from build123d import *

# Parameters (mm, degrees)
SKETCH1_R           = 2
BOSS_EXTRUDE1_DEPTH = 2


with BuildPart() as part:
    # Sketch1 → Boss-Extrude1 (new body)
    with BuildSketch(Plane.XY):
        with BuildLine():
            Line((43.801010204, 68), (43.801010204, 71.053350769))
            ThreePointArc((43.801010204, 71.053350769), (45.533161176, 74.837681982), (49.529475295, 76))
            ThreePointArc((49.529475295, 76), (115.157062367, 0), (49.529475295, -76))
            ThreePointArc((49.529475295, -76), (45.533161176, -74.837681982), (43.801010204, -71.053350769))
            Line((43.801010204, -71.053350769), (43.801010204, -68))
            ThreePointArc((43.801010204, -68), (40.286291578, -59.514718626), (31.801010204, -56))
            Line((31.801010204, -56), (-106.198989796, -56))
            ThreePointArc((-106.198989796, -56), (-126.131547425, 0), (-106.198989796, 56))
            Line((-106.198989796, 56), (31.801010204, 56))
            ThreePointArc((31.801010204, 56), (40.286291578, 59.514718626), (43.801010204, 68))
        make_face()
        with Locations((67, 44)):
            Circle(SKETCH1_R, mode=Mode.SUBTRACT)
        with Locations((67, -44)):
            Circle(SKETCH1_R, mode=Mode.SUBTRACT)
        with Locations((-67, 44)):
            Circle(SKETCH1_R, mode=Mode.SUBTRACT)
        with Locations((-67, -44)):
            Circle(SKETCH1_R, mode=Mode.SUBTRACT)
    extrude(amount=BOSS_EXTRUDE1_DEPTH)


solid = part.part
Build history of the part. All positions in model axes, mm. Coordinates: 2 decimals unless noted, no trailing zeros. Order: outer loops, then holes, each group sorted by start corner. A loop starts at its lowest first (then second) coordinate and runs counter-clockwise, first axis right, second up. Notation, with made-up numbers: (75.5, 64) - (83.5, 64) arc R9 cw to (83.5, 78) - close; hole circle Ø10 at (12.25, -32). An arc over 180 degrees is marked (long way). Write each question's results on one line, items separated by ' | '. Start each with the question number.
Item 1: Band-saw the part on A-A on z = 1.7. Write the cut outline in (x, y).
Item 2: Band-saw the part on C-C on y = 26. Write the cut outline in (x, z).
Item 3: Flat gauge pins, fed straight in: pin 1 (3.5 mm diameter, centred on x = 67, y = -44, fed in from +Z); pin 2 (1 mm diameter, centred on y = 69, z = 1, fed in from -X). Where does each tip first touch, or does it go through?
Item 4: Wall check: probe 1 along Y at (x, z) = (-67, 1.55); probe 2 along X at (y, z) = (1, 1.8); probe 3 along Y at (x, z) = (67, 1). Give the ranges that are in metal, low to high. Write a range as [from, to].
Item 5: Band-saw the part on B-B on x = -40. Write the cut outline in (y, z), and give its area (3 significant figures).
Numbers:
1) outline: (-106.2, -56) - (31.8, -56) arc R12 cw to (43.8, -68) - (43.8, -71.05) arc R5 ccw to (49.53, -76) arc R76.82 ccw to (49.53, 76) arc R5 ccw to (43.8, 71.05) - (43.8, 68) arc R12 cw to (31.8, 56) - (-106.2, 56) arc R88.63 ccw to start; hole circle Ø4 at (-67, -44); hole circle Ø4 at (-67, 44); hole circle Ø4 at (67, -44); hole circle Ø4 at (67, 44)
2) outline: (-122.23, 0) - (110.62, 0) - (110.62, 2) - (-122.23, 2) - close
3) pin 1: through | pin 2: x = 43.8
4) probe 1: [-56, -46], [-42, 42], [46, 56] | probe 2: [-126.13, 115.15] | probe 3: [-71.27, -46], [-42, 42], [46, 71.27]
5) outline: (-56, 0) - (56, 0) - (56, 2) - (-56, 2) - close | area: 224 mm^2
